```python
from build123d import *

# Parameters (mm, degrees)
F0_R     = 21.25
F0_R_2   = 1.65
F0_R_3   = 13
F1_DEPTH = 5
F2_DEPTH = 20
F3_W     = 5
F3_H     = 25
F4_DEPTH = 30
F6_R     = 3.25
F7_DEPTH = 25
F5_R     = 3
F5_R_2   = 3.25
F8_DEPTH = 25
F9_SIZE  = 2.5
F10_R    = 10


# Not quite as in the source:
# - a feature names something its author has since deleted; it is built from what else it names


with BuildPart() as f1:
    # F0 (on Top) → F1 (new body)
    with BuildSketch(Plane.XY):
        with BuildLine():
            Line((30, 60), (5, 60))
            Line((5, 60), (5, 5))
            Line((5, 5), (95, 5))
            Line((95, 5), (95, 59.7859807312))
            ThreePointArc((95, 59.7859807312), (84.7139923095, 92.0261844448), (57.5, 112.1416340365))
            Line((57.5, 112.1416340365), (57.5, 87.5))
            ThreePointArc((57.5, 87.5), (49.4454364826, 68.0545635174), (30, 60))
        make_face()
        with BuildLine():
            Line((40, 120), (5, 120))
            Line((5, 120), (5, 60))
            Line((5, 60), (30, 60))
            ThreePointArc((30, 60), (49.4454364826, 68.0545635174), (57.5, 87.5))
            Line((57.5, 87.5), (57.5, 112.1416340365))
            ThreePointArc((57.5, 112.1416340365), (84.7139923095, 92.0261844448), (95, 59.7859807312))
            Line((95, 59.7859807312), (95, 5))
            Line((95, 5), (100, 5))
            Line((100, 5), (100, 60))
            ThreePointArc((100, 60), (82.4264068712, 102.4264068712), (40, 120))
        make_face()
        with Locations((30, 87)):
            Circle(F0_R, mode=Mode.SUBTRACT)
        with Locations((30, 87)):
            Circle(F0_R)
        with Locations((22.25, 73.5766062413)):
            Circle(F0_R_2, mode=Mode.SUBTRACT)
        with Locations((14.5, 87)):
            Circle(F0_R_2, mode=Mode.SUBTRACT)
        with Locations((37.75, 73.5766062413)):
            Circle(F0_R_2, mode=Mode.SUBTRACT)
        with Locations((30, 87)):
            Circle(F0_R_3, mode=Mode.SUBTRACT)
        with Locations((45.5, 87)):
            Circle(F0_R_2, mode=Mode.SUBTRACT)
        with Locations((22.25, 100.4233937587)):
            Circle(F0_R_2, mode=Mode.SUBTRACT)
        with Locations((37.75, 100.4233937587)):
            Circle(F0_R_2, mode=Mode.SUBTRACT)
        Polygon((0, 120), (0, 0), (100, 0), (100, 5), (95, 5), (5, 5), (5, 60), (5, 120), align=None)
    extrude(amount=F1_DEPTH)

    # F0 (on Top) → F2 (join)
    with BuildSketch(Plane.XY):
        Polygon((0, 120), (0, 0), (100, 0), (100, 5), (95, 5), (5, 5), (5, 60), (5, 120), align=None)
        with BuildLine():
            Line((40, 120), (5, 120))
            Line((5, 120), (5, 60))
            Line((5, 60), (30, 60))
            ThreePointArc((30, 60), (49.4454364826, 68.0545635174), (57.5, 87.5))
            Line((57.5, 87.5), (57.5, 112.1416340365))
            ThreePointArc((57.5, 112.1416340365), (84.7139923095, 92.0261844448), (95, 59.7859807312))
            Line((95, 59.7859807312), (95, 5))
            Line((95, 5), (100, 5))
            Line((100, 5), (100, 60))
            ThreePointArc((100, 60), (82.4264068712, 102.4264068712), (40, 120))
        make_face()
        with Locations((30, 87)):
            Circle(F0_R, mode=Mode.SUBTRACT)
    extrude(amount=-F2_DEPTH)

    # F3 (on face) → F4 (join)
    with BuildSketch(Plane(origin=(0, 120, 0), x_dir=(-1, 0, 0), z_dir=(0, 1, 0))):
        with Locations((-2.5, -7.5)):
            Rectangle(F3_W, F3_H)
    extrude(amount=F4_DEPTH)

    # F6 (on face) → F7 (cut)
    with BuildSketch(Plane.XZ):
        with Locations((22.5, -10)):
            Circle(F6_R)
        with Locations((77.5, -10)):
            Circle(F6_R)
    extrude(amount=-F7_DEPTH, mode=Mode.SUBTRACT)

    # F5 (on face) → F8 (cut)
    with BuildSketch(Plane(origin=(0, 0, 0), x_dir=(0, -1, 0), z_dir=(-1, 0, 0))):
        with Locations((-22.5, -10)):
            Circle(F5_R)
        with Locations((-140, -10)):
            Circle(F5_R_2)
    extrude(amount=-F8_DEPTH, mode=Mode.SUBTRACT)

    # F9
    f9_edges = [f1.edges().sort_by_distance(p)[0] for p in [
        (50, 0, 5),
        (0, 75, 5),
        (0, 0, -7.5),
    ]]
    chamfer(f9_edges, length=F9_SIZE)

    # F10
    f10_edges = [f1.edges().sort_by_distance(p)[0] for p in [
        (5, 5, -10),
        (5, 60, -10),
        (57.5, 112.141634, -10),
        (95, 5, -10),
        (5, 120, -7.5),
        (2.5, 150, -20),
    ]]
    fillet(f10_edges, radius=F10_R)


solid = f1.part
```
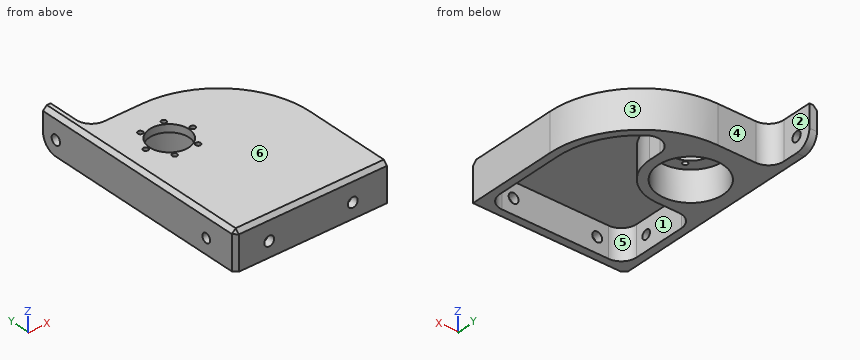
Source: CAD feature listing. Evaluate the final solid. Frame: model axes, mm. Face numbers are marked on the shaded views. A direction names the side the tool comes from. Coordinates: 2 decimals unless noted, no trailing zeros. Write each loop counter-clockwise with the first axis right and the second up, starting at its lowest first coordinate (ties: lowest second). Pieces come first, ordered by that corner, then holes. Notation, with made-up numbers: M 47,71 L 79,71 A21 ccw 79,89 Z; hole C 66,-25.5 d4. An arc over 180 degrees is marked long. Answer as a JSON object with one key per item and string values.
1. Draft query along Y for the marked faces 1, 2 and 3. Return one class per face: released by +Y, released by -Y, zero draft, split by the parting line, or undercut.
Evaluation:
{"face 1": "undercut", "face 2": "zero draft", "face 3": "released by +Y"}
2. Access query for the marked faces 4, 5 and 6. Directions: +Z, -Z, +X, -X, +Y, -Y. A direction counts if a zero-diameter tool reaches every point of the face in a straight line with its end or side. Return the directions, or none.
Evaluation:
{"face 4": "+Z, -Z, +X, +Y", "face 5": "-Z", "face 6": "+Z, +X, -X, +Y, -Y"}
3. Ray query, L1, parallel to Y at x = 30, z = -8.5; L2, parallel to Y at x = 14.5, z = 2.3; L3, parallel to X at y = 42, z = -8.75. Return the intervals inside material, ascending.
Evaluation:
{"L1": "0 to 5, 60 to 65.75, 108.25 to 120", "L2": "0 to 85.35, 88.65 to 120.01", "L3": "0 to 5, 95 to 100"}
4. Cut plane A-A on y = 22.5. Output: boundary loops of the cut face in (x, z).
Evaluation:
{"outline": "M 0,-20 L 5,-20 L 5,-13 L 0,-13 Z; M 0,-7 L 5,-7 L 5,0 L 95,0 L 95,-20 L 100,-20 L 100,5 L 2.5,5 L 0,2.5 Z"}
5. Cut plane B-B on x = 76. Output: boundary loops of the cut face in (y, z), plus the area to 3 significant figures.
Evaluation:
{"outline": "M 0,-20 L 5,-20 L 5,-12.88 L 0,-12.88 Z; M 0,-7.12 L 5,-7.12 L 5,0 L 101.58,0 L 101.58,-20 L 108,-20 L 108,5 L 2.5,5 L 0,2.5 Z", "area": "736 mm^2"}
6. Cut plane C-C on y = 124. Output: boundary loops of the cut face in (x, z), plus the area to 3 significant figures.
Evaluation:
{"outline": "M 0,-20 L 7,-20 L 7,5 L 2.5,5 L 0,2.5 Z", "area": "172 mm^2"}
7. Contact query for flat-ended pins moving along their axis: P1, Ø4, axis at x = 82, y = 45.5, coming from the -Z side; P2, Ø4, axis at y = 90, z = -6.5, coming from the +X side; P3, Ø5, axis at x = 25, z = -1, coming from the +Y side. Output: stop coordinate, or through.
Evaluation:
{"P1": "z = 0", "P2": "x = 93.07", "P3": "y = 120"}
8. Cut plane D-D on x = 61. Output: boundary loops of the cut face in (y, z), plus the area to 3 significant figures.
Evaluation:
{"outline": "M 0,-20 L 5,-20 L 5,0 L 103.22,0 L 103.22,-20 L 116.2,-20 L 116.2,5 L 2.5,5 L 0,2.5 Z", "area": "938 mm^2"}
